Model file for the job. Use its own axes, mm. A direction names the side the tool comes from. Give positions to 0.01 mm unless a question says otherwise; leave off trailing zeros. Write each loop counter-clockwise with the first axis right and the second up, starting at its lowest first coordinate (ties: lowest second). Pieces come first, ordered by that corner, then holes. Notation, with made-up numbers: (-17.5, 41) - (-10.5, 41) arc R20 cw to (-10.5, 60) - close; hole circle Ø6 at (33, -25.5). An arc over 180 degrees is marked (long way). One line per item, written item: value. Start each with the question number.
(1) Drop flat-ended pins along their axis: P1, Ø2.5, axis at x = -11, z = -43, coming from the -Y side; P2, Ø25, axis at y = -82, z = 0, coming from the -X side. Give the stop position or say it passes through.
(2) Probe L1, parallel to X at y = -79, z = -18; L2, parallel to Z at x = 56, y = -32; L3, parallel to Z at x = -65, y = -81. List the from-to ranges inside material, lowest first.
(3) Cut at B-B, the plane z = 0. List the corners of the cut face in (x, y), and give its area (3 significant figures).
(4) 3-axis set-ups, long thin cutter, end or side, ignore diameter. For faces 1 (the face through (39.965, -82, 43)), 2 (the face through (66, -101.6, 1)), 3 (the face through (63.9, -52, -1)): which of +Z, -Z, +X, -X, +Y, -Y reach the whole face in a straight line?
(5) Cut at D-D, the plane x = -51. List the corners of the cut face in (y, z).
(6) Cut at C-C, the plane y = -24.5. List the corners of the cut face in (x, z), and give its area (3 significant figures).
(7) Mould opens along X. For faces 4 (the face through (-39.965, -82, -43)), 5 (the face through (-1, -39, -47.3)), 6 (the face through (71.573, -50, -1)), 7 (the face through (-1, -62.141, -43)) say: pulls with the +X half, pulls with the -X half, needs draft (parallel to the pull), parting line crosses it, or undercut.
(8) Cut at A-A, the plane x = 31. List the corners of the cut face in (y, z).
from build123d import *

# Parameters (mm, degrees)
F0_W     = 143.145382
F0_H     = 94.600484
F1_DEPTH = 101.6
F2_W     = 127.800316
F2_H     = 79.051822
F3_DEPTH = 127
F4_W     = 79.930096
F4_H     = 39.45935
F5_DEPTH = 127
F6_R     = 13.766845
F7_DEPTH = 152.4


with BuildPart() as f1:
    # F0 (on Front) → F1 (new body)
    with BuildSketch(Plane.XZ):
        Rectangle(F0_W, F0_H)
    extrude(amount=F1_DEPTH)

    # F2 (on face) → F3 (cut)
    with BuildSketch(Plane.XZ.offset(101.6)):
        Rectangle(F2_W, F2_H)
    extrude(amount=-F3_DEPTH, mode=Mode.SUBTRACT)

    # F4 (on face) → F5 (cut)
    with BuildSketch(Plane(origin=(0, 0, -47.300242), x_dir=(1, 0, 0), z_dir=(0, 0, -1))):
        with Locations((0, 81.870325)):
            Rectangle(F4_W, F4_H)
    extrude(amount=-F5_DEPTH, mode=Mode.SUBTRACT)

    # F6 (on face) → F7 (cut)
    with BuildSketch(Plane.YZ.offset(71.572691)):
        with Locations((-81.998244, 0)):
            Circle(F6_R)
    extrude(amount=-F7_DEPTH, mode=Mode.SUBTRACT)


solid = f1.part
Answers follow:
1. P1: stops at y = -62.14
1. P2: passes through
2. L1: x = -71.57 to -63.9, 63.9 to 71.57
2. L2: z = -47.3 to -39.53, 39.53 to 47.3
2. L3: z = -47.3 to -13.73, 13.73 to 47.3
3. outline: (-71.57, -101.6) - (-63.9, -101.6) - (-63.9, -95.77) - (-71.57, -95.77) - close; (-71.57, -68.23) - (-63.9, -68.23) - (-63.9, 0) - (-71.57, 0) - close; (63.9, -101.6) - (71.57, -101.6) - (71.57, -95.77) - (63.9, -95.77) - close; (63.9, -68.23) - (71.57, -68.23) - (71.57, 0) - (63.9, 0) - close
3. area: 1,140 mm²
4. face 1: +Z, -Z, -Y
4. face 2: +Z, -Z, +X, -X, -Y
4. face 3: +Y, -Y
5. outline: (-101.6, -47.3) - (0, -47.3) - (0, -39.53) - (-101.6, -39.53) - close; (-101.6, 39.53) - (0, 39.53) - (0, 47.3) - (-101.6, 47.3) - close
6. outline: (-71.57, -47.3) - (71.57, -47.3) - (71.57, 47.3) - (-71.57, 47.3) - close; hole (-63.9, -39.53) - (63.9, -39.53) - (63.9, 39.53) - (-63.9, 39.53) - close
6. area: 3,440 mm²
7. face 4: undercut
7. face 5: needs draft
7. face 6: pulls with the +X half
7. face 7: undercut
8. outline: (-62.14, -47.3) - (0, -47.3) - (0, -39.53) - (-62.14, -39.53) - close; (-62.14, 39.53) - (0, 39.53) - (0, 47.3) - (-62.14, 47.3) - close
